from build123d import *

# Parameters (mm, degrees)
SKETCH1_R                    = 22.225
BOSS_EXTRUDE1_DEPTH          = 0.508
SKETCH2_R                    = 9.525
CUT_EXTRUDE1_DEPTH           = 1.508
F_30_0_1285_DIAMETER_HOLE1_D = 3.2639


with BuildPart() as part:
    # Sketch1 → Boss-Extrude1 (new body)
    with BuildSketch(Plane.XY):
        Circle(SKETCH1_R)
    extrude(amount=BOSS_EXTRUDE1_DEPTH)

    # Sketch2 → Cut-Extrude1 (cut, through all)
    with BuildSketch(Plane.XY.offset(0.508)):
        Circle(SKETCH2_R)
    extrude(amount=-CUT_EXTRUDE1_DEPTH, mode=Mode.SUBTRACT)

    # #30 (0.1285) Diameter Hole1 (through all)
    with Locations(Plane.XY.offset(0.508)):
        with Locations((0, 18.415)):
            f_30_0_1285_diameter_hole1 = Hole(F_30_0_1285_DIAMETER_HOLE1_D / 2)

    # Mirror1: #30 (0.1285) Diameter Hole1 across plane
    add(f_30_0_1285_diameter_hole1.mirror(Plane.ZX), mode=Mode.SUBTRACT)


solid = part.part
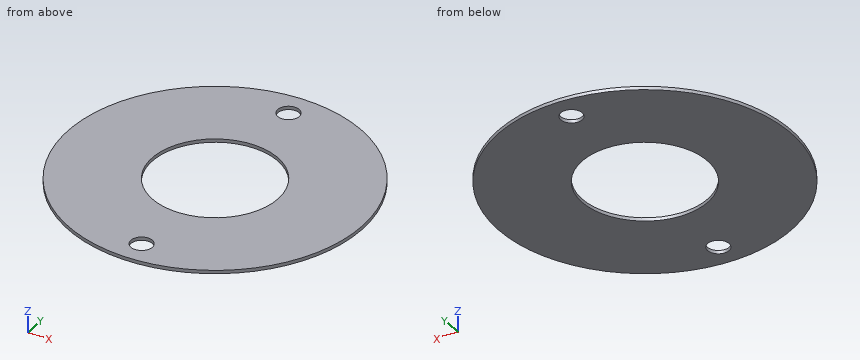
Model file for the job. Use its own axes, mm. Give positions to 0.01 mm unless a question says otherwise; leave off trailing zeros. Order: outer loops, then holes, each group sorted by start corner. A loop starts at its lowest first (then second) coordinate and runs counter-clockwise, first axis right, second up. Notation, with made-up numbers: M 24.5,33 L 82.5,33 A19 ccw 82.5,48 Z; hole C 63.5,40.25 d2. An arc over 180 degrees is marked long. Put each result on its own line as item: value. Start each with the question number.
(1) Band-saw the part on A-A on y = 0. Give the cut face in (x, z) (3 decimals), then the cut area to 3 significant figures.
(2) Band-saw the part on B-B on x = 0. Give the cut face in (y, z) (3 decimals).
(3) Drill centre lines: L1, parallel to Y at x = 0, z = 0.25 (3 decimals); L2, parallel to Y at x = 6.5, z = 0.4; L3, parallel to Y at x = 4, z = 0.1. Where is each one in solid material? Low to high. Write a range as [from, to].
(4) Band-saw the part on C-C on z = 0.4. Give the cut face in (x, y) (3 decimals), then the cut area to 3 significant figures.
(5) Band-saw the part on D-D on x = 11.5. Give the cut face in (y, z).
Results below:
1. outline: M -22.225,0 L -9.525,0 L -9.525,0.508 L -22.225,0.508 Z; M 9.525,0 L 22.225,0 L 22.225,0.508 L 9.525,0.508 Z
1. area: 12.9 mm2
2. outline: M -22.225,0 L -20.047,0 L -20.047,0.508 L -22.225,0.508 Z; M -16.783,0 L -9.525,0 L -9.525,0.508 L -16.783,0.508 Z; M 9.525,0 L 16.783,0 L 16.783,0.508 L 9.525,0.508 Z; M 20.047,0 L 22.225,0 L 22.225,0.508 L 20.047,0.508 Z
3. L1: y = [-22.225, -20.047], [-16.783, -9.525], [9.525, 16.783], [20.047, 22.225]
3. L2: y = [-21.25, -6.96], [6.96, 21.25]
3. L3: y = [-21.86, -8.64], [8.64, 21.86]
4. outline: C 0,0 d44.45; hole C 0,0 d19.05; hole C 0,-18.415 d3.264; hole C 0,18.415 d3.264
4. area: 1,250 mm2
5. outline: M -19.02,0 L 19.02,0 L 19.02,0.51 L -19.02,0.51 Z
